Verification items for the finished model (mm, model axes). A direction names the side the tool comes from. Round coordinates to 2 decimals unless told otherwise and drop trailing zeros. Loops run counter-clockwise (first coordinate to the right, second up) from the corner with the lowest first, then second, coordinate; pieces in that order, holes last. Notation, with made-up numbers: (-29.75, -9) - (22.25, -9) arc R22 ccw to (22.25, 7) - close; hole circle Ø10 at (22, -23.5). An arc over 180 degrees is marked (long way). Use CSV: the item, a comma, the result in double quotes.
```python
from build123d import *

# Parameters (mm, degrees)
SKETCH_1_R          = 75
SKETCH_1_R_2        = 1.25
EXTRUDE_1_DEPTH     = 6
CUT_EXTRUDE_START   = -10
CUT_EXTRUDE_2_DEPTH = 10
CUT_EXTRUDE_3_DEPTH = 10
EXTRUDE_2_DEPTH     = 6
CUT_EXTRUDE_4_DEPTH = 6
SKETCH_8_R          = 2.75
CUT_EXTRUDE_5_DEPTH = 10


with BuildPart() as part:
    # 草图1 → 凸台-拉伸1 (new body)
    with BuildSketch(Plane.XY):
        Circle(SKETCH_1_R)
        with Locations((28.7, -65)):
            Circle(SKETCH_1_R_2, mode=Mode.SUBTRACT)
        with Locations((28.7, -55)):
            Circle(SKETCH_1_R_2, mode=Mode.SUBTRACT)
        with Locations((28.7, -45)):
            Circle(SKETCH_1_R_2, mode=Mode.SUBTRACT)
        with Locations(Location((-28.7, -45, 0), (0, 0, 180))):
            Circle(SKETCH_1_R_2, mode=Mode.SUBTRACT)
        with Locations(Location((-28.7, -55, 0), (0, 0, 180))):
            Circle(SKETCH_1_R_2, mode=Mode.SUBTRACT)
        with Locations(Location((-28.7, -65, 0), (0, 0, 180))):
            Circle(SKETCH_1_R_2, mode=Mode.SUBTRACT)
        with Locations(Location((-24.62114317, 47.354929089, 0), (0, 0, 180))):
            Circle(SKETCH_1_R_2, mode=Mode.SUBTRACT)
        with Locations(Location((-33.281397208, 52.354929089, 0), (0, 0, 180))):
            Circle(SKETCH_1_R_2, mode=Mode.SUBTRACT)
        with Locations(Location((-41.941651246, 57.354929089, 0), (0, 0, 180))):
            Circle(SKETCH_1_R_2, mode=Mode.SUBTRACT)
        with Locations((-53.32114317, -2.354929089)):
            Circle(SKETCH_1_R_2, mode=Mode.SUBTRACT)
        with Locations((-61.981397208, 2.645070911)):
            Circle(SKETCH_1_R_2, mode=Mode.SUBTRACT)
        with Locations((-70.641651246, 7.645070911)):
            Circle(SKETCH_1_R_2, mode=Mode.SUBTRACT)
        with Locations(Location((53.32114317, -2.354929089, 0), (0, 0, 180))):
            Circle(SKETCH_1_R_2, mode=Mode.SUBTRACT)
        with Locations(Location((61.981397208, 2.645070911, 0), (0, 0, 180))):
            Circle(SKETCH_1_R_2, mode=Mode.SUBTRACT)
        with Locations(Location((70.641651246, 7.645070911, 0), (0, 0, 180))):
            Circle(SKETCH_1_R_2, mode=Mode.SUBTRACT)
        with Locations((24.62114317, 47.354929089)):
            Circle(SKETCH_1_R_2, mode=Mode.SUBTRACT)
        with Locations((33.281397208, 52.354929089)):
            Circle(SKETCH_1_R_2, mode=Mode.SUBTRACT)
        with Locations((41.941651246, 57.354929089)):
            Circle(SKETCH_1_R_2, mode=Mode.SUBTRACT)
    extrude(amount=EXTRUDE_1_DEPTH)

    # 草图3 → 切除-拉伸2 (cut)
    with BuildSketch(Plane.XY.offset(6).offset(CUT_EXTRUDE_START)):
        with BuildLine():
            Line((16.2, -37), (16.2, -73.229502251))
            ThreePointArc((16.2, -73.229502251), (0, -75), (-16.2, -73.229502251))
            Line((-16.2, -73.229502251), (-16.2, -37))
            ThreePointArc((-16.2, -37), (-15.614213562, -35.585786438), (-14.2, -35))
            Line((-14.2, -35), (14.2, -35))
            ThreePointArc((14.2, -35), (15.614213562, -35.585786438), (16.2, -37))
        make_face()
        with BuildLine():
            Line((-23.94293994, 32.529611541), (-55.318609256, 50.644362667))
            ThreePointArc((-55.318609256, 50.644362667), (-64.951905284, 37.5), (-71.518609256, 22.585139584))
            Line((-71.518609256, 22.585139584), (-40.14293994, 4.470388459))
            ThreePointArc((-40.14293994, 4.470388459), (-38.62530185, 4.270587614), (-37.410889132, 5.202439266))
            Line((-37.410889132, 5.202439266), (-23.210889132, 29.797560734))
            ThreePointArc((-23.210889132, 29.797560734), (-23.011088287, 31.315198824), (-23.94293994, 32.529611541))
        make_face()
        with BuildLine():
            Line((40.14293994, 4.470388459), (71.518609256, 22.585139584))
            ThreePointArc((71.518609256, 22.585139584), (64.951905284, 37.5), (55.318609256, 50.644362667))
            Line((55.318609256, 50.644362667), (23.94293994, 32.529611541))
            ThreePointArc((23.94293994, 32.529611541), (23.011088287, 31.315198824), (23.210889132, 29.797560734))
            Line((23.210889132, 29.797560734), (37.410889132, 5.202439266))
            ThreePointArc((37.410889132, 5.202439266), (38.62530185, 4.270587614), (40.14293994, 4.470388459))
        make_face()
    extrude(amount=CUT_EXTRUDE_2_DEPTH, mode=Mode.SUBTRACT)

    # 草图5 → 切除-拉伸3 (cut)
    with BuildSketch(Plane.XY.offset(6).offset(CUT_EXTRUDE_START)):
        with BuildLine():
            Line((-40.231963322, 63.296043536), (-6, 43.532210297))
            Line((-6, 43.532210297), (6, 43.532210297))
            Line((6, 43.532210297), (40.231963322, 63.296043536))
            ThreePointArc((40.231963322, 63.296043536), (0, 75), (-40.231963322, 63.296043536))
        make_face()
        with BuildLine():
            Line((74.931963322, 3.193880513), (40.7, -16.569952726))
            Line((40.7, -16.569952726), (34.7, -26.962257571))
            Line((34.7, -26.962257571), (34.7, -66.489924049))
            ThreePointArc((34.7, -66.489924049), (64.951905284, -37.5), (74.931963322, 3.193880513))
        make_face()
        with BuildLine():
            Line((-34.7, -66.489924049), (-34.7, -26.962257571))
            Line((-34.7, -26.962257571), (-40.7, -16.569952726))
            Line((-40.7, -16.569952726), (-74.931963322, 3.193880513))
            ThreePointArc((-74.931963322, 3.193880513), (-64.951905284, -37.5), (-34.7, -66.489924049))
        make_face()
    extrude(amount=CUT_EXTRUDE_3_DEPTH, mode=Mode.SUBTRACT)

    # 草图6 → 凸台-拉伸2 (add)
    with BuildSketch(Plane.XY.offset(6)):
        Polygon((-74.931963322, 3.193880513), (-34.7, -66.489924049), (-34.7, -56.489924049), (-66.271709284, -1.806119487), align=None)
        Polygon((31.571709284, 58.296043536), (40.231963322, 63.296043536), (-40.231963322, 63.296043536), (-31.571709284, 58.296043536), align=None)
        Polygon((34.7, -56.489924049), (34.7, -66.489924049), (74.931963322, 3.193880513), (66.271709284, -1.806119487), align=None)
    extrude(amount=-EXTRUDE_2_DEPTH)

    # 草图7 → 切除-拉伸4 (cut)
    with BuildSketch(Plane.XY.offset(6)):
        Polygon((-25.804939583, -14.898488815), (-10.191166559, -28), (10.191166559, -28), (25.804939583, -14.898488815), (29.344294586, 5.174190865), (19.153128026, 22.825809135), (0, 29.796977629), (-19.153128026, 22.825809135), (-29.344294586, 5.174190865), align=None)
    extrude(amount=-CUT_EXTRUDE_4_DEPTH, mode=Mode.SUBTRACT)

    # 草图8 → 切除-拉伸5 (cut)
    with BuildSketch(Plane.XY.offset(6)):
        with Locations((0, 37.5)):
            Circle(SKETCH_8_R)
        with Locations((32.475952642, -18.75)):
            Circle(SKETCH_8_R)
        with Locations((-32.475952642, -18.75)):
            Circle(SKETCH_8_R)
    extrude(amount=-CUT_EXTRUDE_5_DEPTH, mode=Mode.SUBTRACT)


solid = part.part
```
1) Cross-section at B-B, the plane y = -18.75. Record the cut outline in (x, z), then the cut area to 3 significant figures.
Returned:
outline,"(-62.26, 0) - (-56.49, 0) - (-56.49, 6) - (-62.26, 6) - close; (-39.44, 0) - (-35.23, 0) - (-35.23, 6) - (-39.44, 6) - close; (-29.73, 0) - (-21.21, 0) - (-21.21, 6) - (-29.73, 6) - close; (21.21, 0) - (29.73, 0) - (29.73, 6) - (21.21, 6) - close; (35.23, 0) - (39.44, 0) - (39.44, 6) - (35.23, 6) - close; (56.49, 0) - (62.26, 0) - (62.26, 6) - (56.49, 6) - close"
area,"222 mm²"
2) Cross-section at C-C, the plane y = 15.5. Record the cut outline in (x, z).
Returned:
outline,"(-73.38, 0) - (-59.25, 0) - (-59.25, 6) - (-73.38, 6) - close; (-31.47, 0) - (-23.38, 0) - (-23.38, 6) - (-31.47, 6) - close; (23.38, 0) - (31.47, 0) - (31.47, 6) - (23.38, 6) - close; (59.25, 0) - (73.38, 0) - (73.38, 6) - (59.25, 6) - close"
3) Mould release check, pull along Y, two halves, no side actions. Record for faces 1 (the face through (-1, -34, 0)), 2 (the face through (-48.086, 57.556, 2.958)), 3 (the face through (55.61, 13.4, 2.96)), 4 (the face through (0, -28, 3)): +Y half, -Y half, draft (parallel to the pull), parting line (faces both ways), or undercut.
Returned:
face 1,"draft"
face 2,"+Y half"
face 3,"undercut"
face 4,"undercut"
4) Access from +Z, -Z, +X, -X, +Y, -Y to the whole of each face (thin tool, end or side, straight path). Record for faces 5 (the face through (-39.41, 41.46, 2.96)), 6 (the face through (-55.1, -31.16, 3.04)), 7 (the face through (-18.965, 51.017, 2.958)).
Returned:
face 5,"+Z, -Z, -X"
face 6,"+Z, -Z, -X, -Y"
face 7,"+Z, -Z"
5) Cross-section at D-D, the plane z = 2.5. Count the separate pieces of the cut face and the enclosed holes in it, then the cut area to 3 significant figures.
Returned:
separate pieces,"1"
enclosed holes,"25"
area,"7,540 mm²"
6) Thickness scan on probe 1 along Y at (x, z) = (0, 3.05); probe 2 along X at (y, z) = (-23.5, 5.5); probe 3 along X at (y, z) = (-42, 4.1). Record the ranges inside material, lowest first. Write a range as [from, to].
Returned:
probe 1,"y = [-35, -28], [29.8, 34.75], [40.25, 43.53], [58.3, 63.3]"
probe 2,"x = [-59.52, -53.75], [-36.7, -15.55], [15.55, 36.7], [53.75, 59.52]"
probe 3,"x = [-48.84, -43.07], [-34.7, -16.2], [16.2, 34.7], [43.07, 48.84]"
7) Cross-section at A-A, the plane y = 37.5. Record the cut outline in (x, z).
Returned:
outline,"(-32.55, 0) - (-2.75, 0) - (-2.75, 6) - (-32.55, 6) - close; (2.75, 0) - (32.55, 0) - (32.55, 6) - (2.75, 6) - close"
8) Gauge pin test, flat ends, axial feed: pin 1 Ø1.5 at (x, z) = (23.5, 2) entering from -Y; pin 2 Ø1.5 at (y, z) = (-48.5, 5) entering from -X; pin 3 Ø2 at (y, z) = (-9.5, 4.5) entering from -X. Record the tip position at first contact, or that the pin passes through.
Returned:
pin 1,"stops at y = -71.47"
pin 2,"stops at x = -45.52"
pin 3,"stops at x = -68.18"
